Source: CAD feature listing. Evaluate the final solid. Frame: model axes, mm. A direction names the side the tool comes from. Give positions to 0.01 mm unless a question says otherwise; leave off trailing zeros. Write each loop counter-clockwise with the first axis right and the second up, starting at its lowest first coordinate (ties: lowest second). Pieces come first, ordered by that corner, then holes. Notation, with made-up numbers: (58, 58.5) -> (114, 58.5) arc R23 ccw to (114, 71.5) -> close; hole circle Ø8 at (38, -38). An arc over 180 degrees is marked (long way). Use a Markdown table: item, result. Add a question column.
```python
from build123d import *

# Parameters (mm, degrees)
SKETCH1_W               = 1.984375
SKETCH1_H               = 44.45
SKETCH1_W_2             = 1.5875
SKETCH1_H_2             = 41.275
BOSS_EXTRUDE1_DEPTH     = 3.175
SKETCH11_W              = 1.5875
SKETCH11_H              = 6.769262927
SKETCH11_H_2            = 6.35
BOSS_EXTRUDE2_DEPTH     = 3.175
SKETCHED_START          = -157.95625
SKETCHED_BEND1_DEPTH    = 320.675
SKETCHED_BEND1_2_DEPTH  = 320.675
SKETCHED_START_2        = -28.869188599
SKETCHED_BEND1_3_DEPTH  = 34.81577629
F_3_8_CLEARANCE_HOLE1_D = 10.0838
SKETCH9_W               = 25.908
SKETCH9_H               = 3.683
SKETCH9_W_2             = 25.4
SKETCH9_H_2             = 3.175
CUT_EXTRUDE1_DEPTH      = 176.919307022
SKETCH10_R              = 0.79375
CUT_EXTRUDE2_DEPTH      = 176.919307022


with BuildPart() as part:
    # Sketch1 → Boss-Extrude1 (new body)
    with BuildSketch(Plane(origin=(0, 0, 0), x_dir=(0, 0, -1), z_dir=(1, 0, 0))):
        Polygon((-163.5125, 22.225), (-161.13125, 22.225), (-161.13125, 25.4), (-161.13125, 28.575), (-162.71875, 28.994262927), (-151.928642345, 69.85), (156.36875, 69.85), (156.36875, -69.85), (-151.928642345, -69.85), (-162.71875, -28.994262927), (-161.13125, -28.575), (-161.13125, -25.4), (-161.13125, -22.225), (-163.5125, -22.225), align=None)
        with Locations((157.3609375, 0)):
            Rectangle(SKETCH1_W, SKETCH1_H)
        with Locations((157.1625, -49.2125)):
            Rectangle(SKETCH1_W_2, SKETCH1_H_2)
        with Locations((157.1625, 49.2125)):
            Rectangle(SKETCH1_W_2, SKETCH1_H_2)
    extrude(amount=BOSS_EXTRUDE1_DEPTH)

    # Sketch11 → Boss-Extrude2 (add)
    with BuildSketch(Plane(origin=(3.175, 0, 0), x_dir=(0, 0, -1), z_dir=(1, 0, 0))):
        with Locations((-161.925, 25.609631464)):
            Rectangle(SKETCH11_W, SKETCH11_H)
        with Locations((-161.925, -25.609631464)):
            Rectangle(SKETCH11_W, SKETCH11_H)
        with Locations((157.1625, 25.4)):
            Rectangle(SKETCH11_W, SKETCH11_H_2)
        with Locations((157.1625, -25.4)):
            Rectangle(SKETCH11_W, SKETCH11_H_2)
    extrude(amount=-BOSS_EXTRUDE2_DEPTH)

    # Sketched Bend1: read off the stored shape, not the designer's step
    # Sketched Bend1 outline → Sketched Bend1 (cut)
    with BuildSketch(Plane.XY.offset(SKETCHED_START)):
        with BuildLine():
            Line((2.835373348, 28.70976758), (3.175, 28.994748178))
            Line((3.175, 28.994748178), (3.175, 69.85))
            Line((3.175, 69.85), (0, 69.85))
            Line((0, 69.85), (0, 22.629289812))
            ThreePointArc((0, 22.629289812), (0.74368194, 25.983822265), (2.835373348, 28.70976758))
        make_face()
        with BuildLine():
            Line((3.175, -69.85), (3.175, -28.994748178))
            Line((3.175, -28.994748178), (2.835373348, -28.70976758))
            ThreePointArc((2.835373348, -28.70976758), (0.74368194, -25.983822265), (0, -22.629289812))
            Line((0, -22.629289812), (0, -69.85))
            Line((0, -69.85), (3.175, -69.85))
        make_face()
    extrude(amount=SKETCHED_BEND1_DEPTH, mode=Mode.SUBTRACT)

    # Sketched Bend1 2 outline → Sketched Bend1 2 (add)
    with BuildSketch(Plane.XY.offset(SKETCHED_START)):
        with BuildLine():
            ThreePointArc((3.175, 22.629289812), (3.621209164, 24.642009284), (4.876224009, 26.277576473))
            Line((4.876224009, 26.277576473), (36.804412363, 53.068507545))
            Line((36.804412363, 53.068507545), (34.763561702, 55.500698652))
            Line((34.763561702, 55.500698652), (3.175, 28.994748178))
            Line((3.175, 28.994748178), (3.175, 22.629289812))
        make_face()
        with BuildLine():
            ThreePointArc((4.876224009, -26.277576473), (3.621209164, -24.642009284), (3.175, -22.629289812))
            Line((3.175, -22.629289812), (3.175, -28.994748178))
            Line((3.175, -28.994748178), (34.763561702, -55.500698652))
            Line((34.763561702, -55.500698652), (36.804412363, -53.068507545))
            Line((36.804412363, -53.068507545), (4.876224009, -26.277576473))
        make_face()
    extrude(amount=SKETCHED_BEND1_2_DEPTH)

    # Sketched Bend1 3 outline → Sketched Bend1 3 (cut)
    with BuildSketch(Plane(origin=(0, 0, 0), x_dir=(0, 1, 0), z_dir=(0.9801420201505087, 0, -0.19829679860068306)).offset(SKETCHED_START_2)):
        Polygon((0, 165.039953435), (26.80694597, 160.579525039), (55.500698652, 155.80514942), (57, 155.555679513), (57, 168), (17.789728089, 168), align=None)
        Polygon((-26.80694597, 160.579525039), (0, 165.039953435), (-17.789728089, 168), (-57, 168), (-57, 155.555679513), (-55.500698652, 155.80514942), align=None)
    extrude(amount=SKETCHED_BEND1_3_DEPTH, mode=Mode.SUBTRACT)

    # 3/8 Clearance Hole1 (through all)
    with Locations(Plane(origin=(3.175, 0, 0), x_dir=(0, 0, -1), z_dir=(1, 0, 0))):
        with Locations((115.808125, 0), (26.908125, 0), (-61.991875, 0)):
            Hole(F_3_8_CLEARANCE_HOLE1_D / 2)

    # Sketch9 → Cut-Extrude1 (cut, through all)
    # profile 1 of 4: a face of its own
    with BuildSketch(Plane(origin=(3.175, 0, 0), x_dir=(0, 0, -1), z_dir=(1, 0, 0))):
        with Locations((-125.4125, 18.7325)):
            Rectangle(SKETCH9_W, SKETCH9_H)
        with Locations((-125.4125, 18.7325)):
            Rectangle(SKETCH9_W_2, SKETCH9_H_2, mode=Mode.SUBTRACT)
    # profile 2 of 4: a face of its own
    with BuildSketch(Plane(origin=(3.175, 0, 0), x_dir=(0, 0, -1), z_dir=(1, 0, 0))):
        with Locations((-125.4125, -18.7325)):
            Rectangle(SKETCH9_W, SKETCH9_H)
        with Locations((-125.4125, -18.7325)):
            Rectangle(SKETCH9_W_2, SKETCH9_H_2, mode=Mode.SUBTRACT)
    # profile 3 of 4: a face of its own
    with BuildSketch(Plane(origin=(3.175, 0, 0), x_dir=(0, 0, -1), z_dir=(1, 0, 0))):
        with Locations((120.253125, 18.7325)):
            Rectangle(SKETCH9_W, SKETCH9_H)
        with Locations((120.253125, 18.7325)):
            Rectangle(SKETCH9_W_2, SKETCH9_H_2, mode=Mode.SUBTRACT)
    # profile 4 of 4: a face of its own
    with BuildSketch(Plane(origin=(3.175, 0, 0), x_dir=(0, 0, -1), z_dir=(1, 0, 0))):
        with Locations((120.253125, -18.7325)):
            Rectangle(SKETCH9_W, SKETCH9_H)
        with Locations((120.253125, -18.7325)):
            Rectangle(SKETCH9_W_2, SKETCH9_H_2, mode=Mode.SUBTRACT)
    extrude(amount=-CUT_EXTRUDE1_DEPTH, mode=Mode.SUBTRACT)


with BuildPart() as body_2:
    # of the pieces the cut leaves, the one that is kept (cut_extrude1_keep)
    add(part.part.solids().sort_by_distance((0, 22.225, 163.5125))[0])

    # Sketch10 → Cut-Extrude2 (cut, through all)
    with BuildSketch(Plane(origin=(3.175, 0, 0), x_dir=(0, 0, -1), z_dir=(1, 0, 0))):
        with Locations((108.092875, 16.891)):
            Circle(SKETCH10_R)
        with Locations((108.092875, 20.574)):
            Circle(SKETCH10_R)
        with Locations((132.413375, 20.574)):
            Circle(SKETCH10_R)
        with Locations((132.413375, 16.891)):
            Circle(SKETCH10_R)
        with Locations((132.413375, -16.891)):
            Circle(SKETCH10_R)
        with Locations((132.413375, -20.574)):
            Circle(SKETCH10_R)
        with Locations((108.092875, -20.574)):
            Circle(SKETCH10_R)
        with Locations((108.092875, -16.891)):
            Circle(SKETCH10_R)
        with Locations((-113.25225, -16.891)):
            Circle(SKETCH10_R)
        with Locations((-113.25225, -20.574)):
            Circle(SKETCH10_R)
        with Locations((-137.57275, -20.574)):
            Circle(SKETCH10_R)
        with Locations((-137.57275, -16.891)):
            Circle(SKETCH10_R)
        with Locations((-137.57275, 16.891)):
            Circle(SKETCH10_R)
        with Locations((-137.57275, 20.574)):
            Circle(SKETCH10_R)
        with Locations((-113.25225, 20.574)):
            Circle(SKETCH10_R)
        with Locations((-113.25225, 16.891)):
            Circle(SKETCH10_R)
    extrude(amount=-CUT_EXTRUDE2_DEPTH, mode=Mode.SUBTRACT)


solid = body_2.part
```
(1) Cut plane B-B on x = 26.5. Return the cut outline in (y, z), then the cut area to 3 significant figures.
(2) Cut plane A-A on z = 128.5. Return the cut outline in (x, y) (1 decimal), then the cut area to 3 significant figures.
(3) Material intervals for L1, parallel to X at y = 10, z = -78.5 (3 decimals); L2, parallel to Y at x = 17.5, z = 14; L3, parallel to Y at x = 10, z = -19, sorted ascending.
(4) Cut plane C-C on y = 0. Return the cut outline in (x, z) (1 decimal).
(5) Access query for faces 5 (the flat face through (20.05, -41.22, 157.33)), 6 (the flat face through (2, -26, 162.719)), 7 (the cylindrical face through (0.723, 25.94, 0.137)), 8 (the flat face through (3, 25, 162.719)), 9 (the flat face through (20.62, 39.49, 0.14)). Directions: +Z, -Z, +X, -X, +Y, -Y. A direction counts if a zero-diameter tool reaches every point of the face in a straight line with its end or side. Return the directions, or none.
(6) Mould query, pull axis Y, two halves, no side actions, for faces 1 (the flat face through (20.093, 40.024, 157.524)), 2 (the cylindrical face through (1.565, 0.222, -31.945)), 3 (the cylindrical face through (0.764, -26.028, 0.137)), 4 (the flat face through (21.064, -39.861, 0.137)). Classes: +Y half, -Y half, draft (parallel to the pull), parting line (faces both ways), or undercut.
(7) Cut plane D-D on z = -52. Return the cut outline in (x, y) (1 decimal), then the cut area to 3 significant figures.
(8) First-contact query: pin 1 Ø2.5 at (x, z) = (2, 129.5) entering from +Y; pin 2 Ø10 at (x, y) = (24.5, 42.5) entering from +Z; pin 3 Ø2.5 at (x, z) = (2, -124) entering from -Y; pin 4 Ø9 at (y, z) = (0, -26.91) entering from -X. Flat tips, straight axial feed; report the tip coordinate or a pass-through.
Output:
| question | item | result |
|---|---|---|
| 1 | outline | (-48.57, -157.96) -> (-44.42, -157.96) -> (-44.42, 155.48) -> (-48.57, 154.78) -> close; (44.42, -157.96) -> (48.57, -157.96) -> (48.57, 154.78) -> (44.42, 155.48) -> close |
| 1 | area | 2,600 mm^2 |
| 2 | outline | (0, -22.6) arc R7.9 ccw to (2.8, -28.7) -> (34.8, -55.5) -> (36.8, -53.1) -> (4.9, -26.3) arc R4.8 cw to (3.2, -22.6) -> (3.2, -20.6) -> (0, -20.6) -> close; (0, -16.9) -> (3.2, -16.9) -> (3.2, 16.9) -> (0, 16.9) -> close; (0, 20.6) -> (3.2, 20.6) -> (3.2, 22.6) arc R4.8 cw to (4.9, 26.3) -> (36.8, 53.1) -> (34.8, 55.5) -> (2.8, 28.7) arc R7.9 ccw to (0, 22.6) -> close |
| 2 | area | 420 mm^2 |
| 3 | L1 | 0 to 3.175 |
| 3 | L2 | -41.01 to -36.87, 36.87 to 41.01 |
| 3 | L3 | -34.72 to -30.58, 30.58 to 34.72 |
| 4 | outline | (0, -158.4) -> (3.2, -158.4) -> (3.2, -120.9) -> (0, -120.9) -> close; (0, -110.8) -> (3.2, -110.8) -> (3.2, -32) -> (0, -32) -> close; (0, -21.9) -> (3.2, -21.9) -> (3.2, 56.9) -> (0, 56.9) -> close; (0, 67) -> (3.2, 67) -> (3.2, 163.5) -> (0, 163.5) -> close |
| 5 | face 5 | +Z, +X, -Y |
| 5 | face 6 | +Z, +X, -X, -Y |
| 5 | face 7 | +Z, -Z, -X, +Y |
| 5 | face 8 | +Z, +X, -X, +Y |
| 5 | face 9 | +Z, -Z, +X |
| 6 | face 1 | +Y half |
| 6 | face 2 | undercut |
| 6 | face 3 | -Y half |
| 6 | face 4 | undercut |
| 7 | outline | (0, -22.6) arc R7.9 ccw to (2.8, -28.7) -> (34.8, -55.5) -> (36.8, -53.1) -> (4.9, -26.3) arc R4.8 cw to (3.2, -22.6) -> (3.2, 22.6) arc R4.8 cw to (4.9, 26.3) -> (36.8, 53.1) -> (34.8, 55.5) -> (2.8, 28.7) arc R7.9 ccw to (0, 22.6) -> close |
| 7 | area | 444 mm^2 |
| 8 | pin 1 | y = 29.06 |
| 8 | pin 2 | z = 157.53 |
| 8 | pin 3 | y = -29.06 |
| 8 | pin 4 | through |
